from build123d import *

# Parameters (mm, degrees)
SKETCH1_W           = 5
SKETCH1_H           = 80
BOSS_EXTRUDE1_DEPTH = 80


with BuildPart() as part:
    # Sketch1 → Revolve1 (revolve)
    with BuildSketch(Plane.XY, mode=Mode.PRIVATE) as revolve1_sk:
        with Locations((-2.5, -40)):
            Rectangle(SKETCH1_W, SKETCH1_H)
    revolve(revolve1_sk.sketch.rotate(Axis((0, 80, 0), (0, -1, 0)), 270), axis=Axis((0, 80, 0), (0, -1, 0)))

    # Sketch2 → Boss-Extrude1 (add)
    with BuildSketch(Plane(origin=(0, 0, 0), x_dir=(1, 0, 0), z_dir=(0, 1, 0))):
        with BuildLine():
            Line((-0.5, 3.464101615), (0, 5))
            Line((0, 5), (0.5, 3.464101615))
            ThreePointArc((0.5, 3.464101615), (0.727690918, 3.423516603), (0.952204333, 3.367982617))
            Line((0.952204333, 3.367982617), (2.033683215, 4.567727288))
            Line((2.033683215, 4.567727288), (1.865749791, 2.961245974))
            ThreePointArc((1.865749791, 2.961245974), (2.057248383, 2.83155948), (2.239763887, 2.689508827))
            Line((2.239763887, 2.689508827), (3.715724127, 3.345653032))
            Line((3.715724127, 3.345653032), (2.908894493, 1.946364001))
            ThreePointArc((2.908894493, 1.946364001), (3.031088913, 1.75), (3.140047917, 1.545994527))
            Line((3.140047917, 1.545994527), (4.755282581, 1.545084972))
            Line((4.755282581, 1.545084972), (3.449064911, 0.594938011))
            ThreePointArc((3.449064911, 0.594938011), (3.480826634, 0.365849621), (3.497389136, 0.135163729))
            Line((3.497389136, 0.135163729), (4.972609477, -0.522642316))
            Line((4.972609477, -0.522642316), (3.392860672, -0.859358166))
            ThreePointArc((3.392860672, -0.859358166), (3.328697807, -1.08155948), (3.25, -1.299038106))
            Line((3.25, -1.299038106), (4.330127019, -2.5))
            Line((4.330127019, -2.5), (2.75, -2.165063509))
            ThreePointArc((2.75, -2.165063509), (2.601006889, -2.341957122), (2.440656339, -2.508624451))
            Line((2.440656339, -2.508624451), (2.938926261, -4.045084972))
            Line((2.938926261, -4.045084972), (1.631639345, -3.096409703))
            ThreePointArc((1.631639345, -3.096409703), (1.423578251, -3.197409102), (1.209301024, -3.284446838))
            Line((1.209301024, -3.284446838), (1.039558454, -4.890738004))
            Line((1.039558454, -4.890738004), (0.231153424, -3.492358529))
            ThreePointArc((0.231153424, -3.492358529), (0, -3.5), (-0.231153424, -3.492358529))
            Line((-0.231153424, -3.492358529), (-1.039558454, -4.890738004))
            Line((-1.039558454, -4.890738004), (-1.209301024, -3.284446838))
            ThreePointArc((-1.209301024, -3.284446838), (-1.423578251, -3.197409102), (-1.631639345, -3.096409703))
            Line((-1.631639345, -3.096409703), (-2.938926261, -4.045084972))
            Line((-2.938926261, -4.045084972), (-2.440656339, -2.508624451))
            ThreePointArc((-2.440656339, -2.508624451), (-2.601006889, -2.341957122), (-2.75, -2.165063509))
            Line((-2.75, -2.165063509), (-4.330127019, -2.5))
            Line((-4.330127019, -2.5), (-3.25, -1.299038106))
            ThreePointArc((-3.25, -1.299038106), (-3.328697807, -1.08155948), (-3.392860672, -0.859358166))
            Line((-3.392860672, -0.859358166), (-4.972609477, -0.522642316))
            Line((-4.972609477, -0.522642316), (-3.497389136, 0.135163729))
            ThreePointArc((-3.497389136, 0.135163729), (-3.480826634, 0.365849621), (-3.449064911, 0.594938011))
            Line((-3.449064911, 0.594938011), (-4.755282581, 1.545084972))
            Line((-4.755282581, 1.545084972), (-3.140047917, 1.545994527))
            ThreePointArc((-3.140047917, 1.545994527), (-3.031088913, 1.75), (-2.908894493, 1.946364001))
            Line((-2.908894493, 1.946364001), (-3.715724127, 3.345653032))
            Line((-3.715724127, 3.345653032), (-2.239763887, 2.689508827))
            ThreePointArc((-2.239763887, 2.689508827), (-2.057248383, 2.83155948), (-1.865749791, 2.961245974))
            Line((-1.865749791, 2.961245974), (-2.033683215, 4.567727288))
            Line((-2.033683215, 4.567727288), (-0.952204333, 3.367982617))
            ThreePointArc((-0.952204333, 3.367982617), (-0.727690918, 3.423516603), (-0.5, 3.464101615))
        make_face()
    extrude(amount=BOSS_EXTRUDE1_DEPTH)


solid = part.part
Source: CAD feature listing. Evaluate the final solid. Frame: model axes, mm. Give positions to 0.01 mm unless a question says otherwise; leave off trailing zeros. Order: outer loops, then holes, each group sorted by start corner. A loop starts at its lowest first (then second) coordinate and runs counter-clockwise, first axis right, second up. Notation, with made-up numbers: (-4.5, -28.5) -> (4.5, -28.5) arc R23 cw to (4.5, 5.5) -> close; hole circle Ø2 at (-7.5, 8.5). An arc over 180 degrees is marked (long way). Write item = value, one per line.
Q1. Material intervals for line 1 (Z direction, x = -4, y = 54); line 2 (X direction, y = 33, z = -4); line 3 (X direction, y = 57, z = -0.25), sorted ascending. Write a range as from..to.
Data:
line_1 = -1.55..-1, 0.09..0.73, 2.13..2.43
line_2 = -1.97..-1.52, -0.33..0.33, 1.52..1.97
line_3 = -3.49..3.49
Q2. Pin query (flat end, axial travel): pin 1 (4 mm diameter, centred on y = 36.5, z = 0.5, fed in from -X); pin 2 (0.9 mm diameter, centred on x = 4, z = 3, fed in from +Y); pin 3 (2 mm diameter, centred on y = -50.5, z = -3.5, fed in from +X). Return the tip coordinate at first contact, or that it passes through.
Data:
pin_1 = -4.97
pin_2 = 0
pin_3 = 4.33
Q3. Cut plane A-A, the plane y = -17.5. Output: boundary loops of the cut face in (x, z).
Data:
outline = circle Ø10 at (0, 0)
